Source: CAD feature listing. Evaluate the final solid. Frame: model axes, mm. A direction names the side the tool comes from. Give positions to 0.01 mm unless a question says otherwise; leave off trailing zeros. Loops run counter-clockwise (first coordinate to the right, second up) from the corner with the lowest first, then second, coordinate; pieces in that order, holes last. Notation, with made-up numbers: (8, 86) - (62, 86) arc R10 cw to (62, 96) - close; hole circle Ø9 at (31.5, 14). An arc over 180 degrees is marked (long way). Write each question's results on one line, items separated by ' | '. Start each with the question number.
(1) Cut plane D-D on y = 18.5. Return the cut outline in (x, z), then the cut area to 3 significant figures.
(2) Cut plane C-C on z = -3.5. Return the cut outline in (x, y), then the cut area to 3 significant figures.
(3) Cut plane B-B on x = -6. Return the cut outline in (y, z).
(4) Cut plane A-A on y = 0. Return the cut outline in (x, z).
(5) Contact query for flat-ended pins moving along their axis: pin 1 (3 mm diameter, centred on x = -50, y = 2.5, fed in from +Z); pin 2 (1 mm diameter, centred on x = -2.5, y = 12.5, fed in from -Z); pin 3 (4 mm diameter, centred on y = 27.5, z = 23, fed in from -X). Output: stop coordinate, or through.
(6) Pull-direction query (X, two-part tool) for faces 1 (the cylindrical face through (-36.073, 28.154, 8.274)), 2 (the flat face through (-47.85, -20.02, 4.93)); classes: pulls with the +X half, pulls with the -X half, needs draft (parallel to the pull), parting line crosses it, or undercut.
(7) Material intervals for line 1 along Y through (x, z) = (-35, 3); line 2 along Y through (x, z) = (22, 2); line 3 along Z through (x, y) = (-56, 10), sorted ascending. Write a range as [from, to].
(8) Reachability of faces 3 (the cylindrical face through (-60.58, 14.56, 4.93)), 4 (the cylindrical face through (22.74, 29.58, 3.2)), 5 (the cylindrical face through (-65, 0, 5)), 6 (the flat face through (17.825, 33.476, 4.93)), 7 (the flat face through (-21.54, 28.248, 8.274)) from +Z, -Z, +X, -X, +Y, -Y: full face, straight path, thin tool, end or side. Return the list, or none.
from build123d import *

# Parameters (mm, degrees)
ESQUISSE1_R             = 1.6
BOSS_EXTRU_1_DEPTH      = 10
ESQUISSE2_R             = 32.8
BOSS_EXTRU_2_DEPTH      = 22
ENL_V_MAT_EXTRU_1_DEPTH = 3.5
BOSS_EXTRU_3_REACH      = 12
ESQUISSE4_R             = 32.8
ESQUISSE5_R             = 16
BOSS_EXTRU_4_DEPTH      = 19
ESQUISSE8_R             = 5
BOSS_EXTRU_7_DEPTH      = 5.5


with BuildPart() as part:
    # Esquisse1 → Boss.-Extru.1 (new body)
    with BuildSketch(Plane.XY):
        with BuildLine():
            ThreePointArc((-56.3, -16.861494596), (-60.528670487, -14.599558136), (-64.01, -11.301322931))
            ThreePointArc((-64.01, -11.301322931), (-65, 0), (-64.01, 11.301322931))
            ThreePointArc((-64.01, 11.301322931), (-60.528670487, 14.599558136), (-56.3, 16.861494596))
            Line((-56.3, 16.861494596), (-39.624688626, 23.091930519))
            ThreePointArc((-39.624688626, 23.091930519), (-36.690940127, 29.525679018), (-30.257191628, 26.591930519))
            Line((-30.257191628, 26.591930519), (-12.425, 33.254614341))
            ThreePointArc((-12.425, 33.254614341), (1.381675102, 35.473102119), (14.973963383, 32.187426436))
            Line((14.973963383, 32.187426436), (20.756023105, 34.801647207))
            ThreePointArc((20.756023105, 34.801647207), (24.347774736, 34.238511045), (26, 31))
            Line((26, 31), (25.359978077, 24.841930519))
            ThreePointArc((25.359978077, 24.841930519), (35.5, 0), (25.359978077, -24.841930519))
            Line((25.359978077, -24.841930519), (26, -31))
            ThreePointArc((26, -31), (24.347774736, -34.238511045), (20.756023105, -34.801647207))
            Line((20.756023105, -34.801647207), (14.973963383, -32.187426436))
            ThreePointArc((14.973963383, -32.187426436), (1.381675102, -35.473102119), (-12.425, -33.254614341))
            Line((-12.425, -33.254614341), (-30.257191628, -26.591930519))
            ThreePointArc((-30.257191628, -26.591930519), (-36.690940127, -29.525679018), (-39.624688626, -23.091930519))
            Line((-39.624688626, -23.091930519), (-56.3, -16.861494596))
        make_face()
        with Locations((-35, -25)):
            Circle(ESQUISSE1_R, mode=Mode.SUBTRACT)
        with Locations((22, 31)):
            Circle(ESQUISSE1_R, mode=Mode.SUBTRACT)
        with Locations((-35, 25)):
            Circle(ESQUISSE1_R, mode=Mode.SUBTRACT)
        with Locations((22, -31)):
            Circle(ESQUISSE1_R, mode=Mode.SUBTRACT)
    extrude(amount=BOSS_EXTRU_1_DEPTH)

    # Esquisse2 → Boss.-Extru.2 (add)
    with BuildSketch(Plane.XY.offset(10)):
        Circle(ESQUISSE2_R)
    extrude(amount=BOSS_EXTRU_2_DEPTH)

    # Esquisse3 → Enlèv. mat.-Extru.1 (cut)
    with BuildSketch(Plane.XY.offset(10)):
        with BuildLine():
            Line((-55.775, -15.456370046), (-37.378202776, -22.330008789))
            ThreePointArc((-37.378202776, -22.330008789), (-36.165940127, -28.120554469), (-31.453677478, -24.543603151))
            Line((-31.453677478, -24.543603151), (-11.9, -31.849489792))
            ThreePointArc((-11.9, -31.849489792), (1.664031028, -33.959255009), (14.956816294, -30.533484019))
            Line((14.956816294, -30.533484019), (21.291141631, -33.397398551))
            ThreePointArc((21.291141631, -33.397398551), (23.468656713, -33.023128137), (24.499056843, -31.06866508))
            Line((24.499056843, -31.06866508), (23.79417774, -24.286562245))
            ThreePointArc((23.79417774, -24.286562245), (34, 0), (23.79417774, 24.286562245))
            Line((23.79417774, 24.286562245), (24.499056843, 31.06866508))
            ThreePointArc((24.499056843, 31.06866508), (23.468656713, 33.023128137), (21.291141631, 33.397398551))
            Line((21.291141631, 33.397398551), (14.956816294, 30.533484019))
            ThreePointArc((14.956816294, 30.533484019), (1.664031028, 33.959255009), (-11.9, 31.849489792))
            Line((-11.9, 31.849489792), (-31.453677478, 24.543603151))
            ThreePointArc((-31.453677478, 24.543603151), (-36.165940127, 28.120554469), (-37.378202776, 22.330008789))
            Line((-37.378202776, 22.330008789), (-55.775, 15.456370046))
            ThreePointArc((-55.775, 15.456370046), (-59.496201473, 13.493411636), (-62.6, 10.653168543))
            ThreePointArc((-62.6, 10.653168543), (-63.5, 0), (-62.6, -10.653168543))
            ThreePointArc((-62.6, -10.653168543), (-59.496201473, -13.493411636), (-55.775, -15.456370046))
        make_face()
    extrude(amount=-ENL_V_MAT_EXTRU_1_DEPTH, mode=Mode.SUBTRACT)

    # Esquisse4 → Boss.-Extru.3 (add, up to next)
    with BuildSketch(Plane(origin=(0, 0, 10), x_dir=(-1, 0, 0), z_dir=(0, 0, -1)), mode=Mode.PRIVATE) as boss_extru_3_sk1:
        Circle(ESQUISSE4_R)
    boss_extru_3_tool1 = extrude(boss_extru_3_sk1.sketch, amount=BOSS_EXTRU_3_REACH, mode=Mode.PRIVATE) - part.part
    add(boss_extru_3_tool1.solids().sort_by_distance((0, 0, 10))[0])

    # Esquisse5 → Boss.-Extru.4 (add)
    with BuildSketch(Plane(origin=(0, 0, 0), x_dir=(-1, 0, 0), z_dir=(0, 0, -1))):
        with Locations((50, 0)):
            Circle(ESQUISSE5_R)
    extrude(amount=BOSS_EXTRU_4_DEPTH)

    # Esquisse8 → Boss.-Extru.7 (add)
    with BuildSketch(Plane.XY.offset(6.5)):
        with Locations((-50, 0)):
            Circle(ESQUISSE8_R)
    extrude(amount=BOSS_EXTRU_7_DEPTH)


solid = part.part
Ans:
1) outline: (-51.91, 0) - (30.3, 0) - (30.3, 10) - (28.53, 10) - (28.53, 6.5) - (27.08, 6.5) - (27.08, 32) - (-27.08, 32) - (-27.08, 6.5) - (-47.63, 6.5) - (-47.63, 10) - (-51.91, 10) - close | area: 1,940 mm^2
2) outline: circle Ø32 at (-50, 0) | area: 804 mm^2
3) outline: (-34.99, 0) - (34.99, 0) - (34.99, 10) - (33.47, 10) - (33.47, 6.5) - (32.25, 6.5) - (32.25, 32) - (-32.25, 32) - (-32.25, 6.5) - (-33.47, 6.5) - (-33.47, 10) - (-34.99, 10) - close
4) outline: (-66, -19) - (-34, -19) - (-34, 0) - (35.5, 0) - (35.5, 10) - (34, 10) - (34, 6.5) - (32.8, 6.5) - (32.8, 32) - (-32.8, 32) - (-32.8, 6.5) - (-45, 6.5) - (-45, 12) - (-55, 12) - (-55, 6.5) - (-63.5, 6.5) - (-63.5, 10) - (-65, 10) - (-65, 0) - (-66, 0) - close
5) pin 1: z = 12 | pin 2: z = 0 | pin 3: x = -20.63
6) face 1: undercut | face 2: pulls with the -X half
7) line 1: [-29.84, -26.6], [-23.4, 23.4], [26.6, 29.84] | line 2: [-35, -32.6], [-29.4, 29.4], [32.6, 35] | line 3: [-19, 6.5]
8) face 3: +Z, -Z, -X, +Y | face 4: +Z, -Z | face 5: +Z, -X | face 6: +Z, -Z, +Y | face 7: +Z
